```python
from build123d import *

# Parameters (mm, degrees)
SKETCH2_R           = 50
SKETCH2_R_2         = 15
BOSS_EXTRUDE1_DEPTH = 90
BOSS_EXTRUDE2_START = -90
BOSS_EXTRUDE2_DEPTH = 90
SKETCH4_R           = 15
BOSS_EXTRUDE3_DEPTH = 25


with BuildPart() as part:
    # Sketch2 → Boss-Extrude1 (new body)
    with BuildSketch(Plane(origin=(0, 0, 0), x_dir=(1, 0, 0), z_dir=(0, 1, 0))):
        with Locations(Location((0, 0, 0), (0, 0, 90))):
            Circle(SKETCH2_R)
        with Locations(Location((0, 0, 0), (0, 0, 90))):
            Circle(SKETCH2_R_2, mode=Mode.SUBTRACT)
    extrude(amount=BOSS_EXTRUDE1_DEPTH)

    # Sketch3 → Boss-Extrude2 (add)
    with BuildSketch(Plane(origin=(0, 90, 0), x_dir=(1, 0, 0), z_dir=(0, 1, 0)).offset(BOSS_EXTRUDE2_START)):
        with BuildLine():
            Line((-50, 0), (-50, 125))
            Line((-50, 125), (50, 125))
            Line((50, 125), (50, 0))
            ThreePointArc((50, 0), (0, 50), (-50, 0))
        make_face()
    extrude(amount=BOSS_EXTRUDE2_DEPTH)

    # Sketch4 → Boss-Extrude3 (add)
    with BuildSketch(Plane(origin=(0, 0, -125), x_dir=(-1, 0, 0), z_dir=(0, 0, -1))):
        with Locations((0, 47.976232204)):
            Circle(SKETCH4_R)
    extrude(amount=BOSS_EXTRUDE3_DEPTH)


solid = part.part
```
Model file for the job. Use its own axes, mm. A direction names the side the tool comes from. Coordinates: 2 decimals unless noted, no trailing zeros. Loops run counter-clockwise (first coordinate to the right, second up) from the corner with the lowest first, then second, coordinate; pieces in that order, holes last. Notation, with made-up numbers: (5, 16) -> (31, 16) arc R27 ccw to (31, 54) -> close; hole circle Ø9 at (7, 78). An arc over 180 degrees is marked (long way). Answer as a JSON object with one key per item and string values.
Q1. Flat gauge pins, fed straight in: P1, Ø4, axis at x = -27, y = 35.5, coming from the +Z side; P2, Ø8, axis at x = 25, y = 62.5, coming from the +Z side; P3, Ø1.5, axis at y = 72.5, z = 26.5, coming from the -X side. Where does each tip first touch, or does it go through?
Report:
{"P1": "stops at z = 43.3", "P2": "stops at z = 45.38", "P3": "stops at x = -42.86"}
Q2. Probe probe 1 along Z at (x, y) = (-1, 48.5); probe 2 along X at (y, z) = (40, 0); probe 3 along Z at (x, y) = (12, 34.5). List the from-to ranges inside material, lowest first.
Report:
{"probe 1": "z = -150 to -14.97, 14.97 to 49.99", "probe 2": "x = -50 to -15, 15 to 50", "probe 3": "z = -125 to -9, 9 to 48.54"}
Q3. Cut at B-B (y = 59.5). List the corners of the cut face in (x, z).
Report:
{"outline": "(-50, -125) -> (-9.6, -125) -> (-9.6, -150) -> (9.6, -150) -> (9.6, -125) -> (50, -125) -> (50, 0) arc R50 ccw to (-50, 0) -> close; hole circle Ø30 at (0, 0)"}
Q4. Cut at C-C (z = 2). List the corners of the cut face in (x, y).
Report:
{"outline": "(-49.96, 0) -> (-14.87, 0) -> (-14.87, 90) -> (-49.96, 90) -> close; (14.87, 0) -> (49.96, 0) -> (49.96, 90) -> (14.87, 90) -> close"}
Q5. Cut at D-D (y = 42.5). List the corners of the cut face in (x, z), and give its area (3 significant figures).
Report:
{"outline": "(-50, -125) -> (-13.96, -125) -> (-13.96, -150) -> (13.96, -150) -> (13.96, -125) -> (50, -125) -> (50, 0) arc R50 ccw to (-50, 0) -> close; hole circle Ø30 at (0, 0)", "area": "16,400 mm2"}
Q6. Pull direction X, two halves, no side cores. Call faces 1 (the flat face through (1, 90, -39)), 2 (the cylindrical face through (-1.099, 44.37, 49.988)), 3 (the cylindrical face through (-0.66, 44.37, 14.985)): released by +X, released by -X, zero draft, split by the parting line, or undercut.
Report:
{"face 1": "zero draft", "face 2": "split by the parting line", "face 3": "undercut"}
Q7. 3-axis set-ups, long thin cutter, end or side, ignore diameter. For faces 4 (the flat face through (-12, 34, -125)), 5 (the flat face through (0, 48, -150)): which of +Z, -Z, +X, -X, +Y, -Y reach the whole face in a straight line?
Report:
{"face 4": "-Z", "face 5": "-Z, +X, -X, +Y, -Y"}
Q8. Cut at A-A (x = 0). List the corners of the cut face in (y, z), and give its area (3 significant figures).
Report:
{"outline": "(0, -125) -> (32.98, -125) -> (32.98, -150) -> (62.98, -150) -> (62.98, -125) -> (90, -125) -> (90, -15) -> (0, -15) -> close; (0, 15) -> (90, 15) -> (90, 50) -> (0, 50) -> close", "area": "13,800 mm2"}
